Part model, mm, in its own coordinate system. A direction names the side the tool comes from. Give positions to 0.01 mm unless a question says otherwise; leave off trailing zeros. Write each loop counter-clockwise with the first axis right and the second up, starting at its lowest first coordinate (ties: lowest second). Pieces come first, ordered by that corner, then holes. Notation, with made-up numbers: M 38,31.5 L 69,31.5 A15 ccw 69,40.5 Z; hole C 18,-10 d3. An arc over 180 degrees is marked long. Write item = value, one per line. Start each with the question number.
from build123d import *

# Parameters (mm, degrees)
F1_DEPTH = 76.2
F3_DEPTH = 1.27
F5_DEPTH = 1.27


with BuildPart() as f1:
    # F0 (on Right) → F1 (new body, symmetric)
    with BuildSketch(Plane.YZ):
        Polygon((26.177771, 39.065287), (-3.893106, 0), (26.177771, 0), (45.777533, 0), (45.777533, 39.065287), align=None)
    extrude(amount=F1_DEPTH, both=True)

    # F2 (on face) → F3 (join)
    with BuildSketch(Plane.YZ.offset(76.2)):
        Polygon((-10.503355, 5.088302), (-3.893106, 0), (26.177771, 39.065287), (19.567522, 44.153589), align=None)
    extrude(amount=-F3_DEPTH)

    # F4 (on face) → F5 (join)
    with BuildSketch(Plane(origin=(-76.2, 0, 0), x_dir=(0, -1, 0), z_dir=(-1, 0, 0))):
        Polygon((-19.752756, 44.011004), (-26.177771, 39.065287), (3.893106, 0), (10.318121, 4.945717), align=None)
    extrude(amount=-F5_DEPTH)


solid = f1.part
Q1. Slice it at D-D (y = 29). Give the cut face in (x, z).
Q2. Probe line 1 along X through (y, z) = (16, 37); line 2 along Z through (x, y) = (-63, 38.5); line 3 along Z through (x, y) = (-6, 0). List the from-to ranges inside material, lowest first.
Q3. Slice it at C-C (x = 52). Give the cut face in (y, z), and give its area (3 significant figures).
Q4. Drop flat-ended pins along their axis: P1, Ø10, axis at x = 48, z = 21.5, coming from the -Y side; P2, Ø1.5, axis at x = -56, y = 24, coming from the +Z side; P3, Ø6, axis at x = 35.5, y = 7, coming from the -Z side; P4, Ø15.5, axis at x = -28.5, y = 34, coming from the +Z side. Give the stop position or say it passes through.
Q5. Tool access for faces 5 (the face through (-75.574, 4.507, 24.205)), 6 (the face through (-74.93, 7, 22)), 7 (the face through (-75.57, -7.06, 2.44)): list every direction of +Z, -Z, +X, -X, +Y, -Y with a clear straight run to the whole face (end or side of a thin tool).
Q6. Two-plate mould, pull along X, no slides. Class faces 1 (the face through (-76.2, 24, 17)), 2 (the face through (1.049, 11.353, 19.806)), 3 (the face through (74.93, 6, 22)), 4 (the face through (76.2, 23, 17)): +X half, -X half, draft (parallel to the pull), parting line (faces both ways), or undercut.
Q7. Slice it at A-A (z = 16). Give the cut face in (x, y).
Q8. Slice it at B-B (y = 15). Give the cut face in (x, z).
Working result:
q1.outline = M -76.2,0 L 76.2,0 L 76.2,39.07 L -76.2,39.07 Z
q2.line_1 = -76.2 to -74.93, 74.93 to 76.2
q2.line_2 = 0 to 39.07
q2.line_3 = 0 to 5.06
q3.outline = M -3.89,0 L 45.78,0 L 45.78,39.07 L 26.18,39.07 Z
q3.area = 1,350 mm2
q4.P1 = 8.81
q4.P2 = 37.21
q4.P3 = 0
q4.P4 = 39.07
q5.face_5 = +Z, -X, -Y
q5.face_6 = +Z, -Y
q5.face_7 = -Z, +X, -X, -Y
q6.face_1 = -X half
q6.face_2 = undercut
q6.face_3 = undercut
q6.face_4 = +X half
q7.outline = M -76.2,-1.81 L -74.93,-1.81 L -74.93,8.42 L 74.93,8.42 L 74.93,-2.1 L 76.2,-2.1 L 76.2,45.78 L -76.2,45.78 Z
q8.outline = M -76.2,0 L 76.2,0 L 76.2,38.22 L 74.93,38.22 L 74.93,24.54 L -74.93,24.54 L -74.93,37.84 L -76.2,37.84 Z
